Verification items for the finished model (mm, model axes). Round coordinates to 2 decimals unless told otherwise and drop trailing zeros. Write each loop counter-clockwise with the first axis right and the second up, starting at its lowest first coordinate (ties: lowest second). Pieces come first, ordered by that corner, then holes. Notation, with made-up numbers: M 77.5,68 L 83.5,68 A25 ccw 83.5,98 Z; hole C 43.25,-36 d4. An arc over 180 degrees is marked long. Use a Markdown table: item, result. Add a question column.
from build123d import *

# Parameters (mm, degrees)
ESQUISSE1_W             = 520
ESQUISSE1_H             = 42
BOSS_EXTRU_1_DEPTH      = 15
ESQUISSE2_R             = 10.5
ENL_V_MAT_EXTRU_1_DEPTH = 15
ESQUISSE3_W             = 10
ESQUISSE3_H             = 42
ENL_V_MAT_EXTRU_2_DEPTH = 262.277630118
ESQUISSE4_W             = 345
ESQUISSE4_H             = 5
ENL_V_MAT_EXTRU_3_DEPTH = 2


with BuildPart() as part:
    # Esquisse1 → Boss.-Extru.1 (new body)
    with BuildSketch(Plane(origin=(0, 0, 0), x_dir=(1, 0, 0), z_dir=(0, 1, 0))):
        Rectangle(ESQUISSE1_W, ESQUISSE1_H)
    extrude(amount=BOSS_EXTRU_1_DEPTH)

    # Esquisse2 → Enlèv. mat.-Extru.1 (cut)
    with BuildSketch(Plane(origin=(0, 15, 0), x_dir=(1, 0, 0), z_dir=(0, 1, 0))):
        with Locations(Location((-229, 0, 0), (0, 0, 270))):
            Circle(ESQUISSE2_R)
        with Locations(Location((229, 0, 0), (0, 0, 270))):
            Circle(ESQUISSE2_R)
    extrude(amount=-ENL_V_MAT_EXTRU_1_DEPTH, mode=Mode.SUBTRACT)

    # Esquisse3 → Enlèv. mat.-Extru.2 (cut, through all)
    with BuildSketch(Plane(origin=(0, 15, 0), x_dir=(1, 0, 0), z_dir=(0, 1, 0))):
        with Locations((-255, 0)):
            Rectangle(ESQUISSE3_W, ESQUISSE3_H)
        with Locations((255, 0)):
            Rectangle(ESQUISSE3_W, ESQUISSE3_H)
    extrude(amount=-ENL_V_MAT_EXTRU_2_DEPTH, mode=Mode.SUBTRACT)

    # Esquisse4 → Enlèv. mat.-Extru.3 (cut)
    with BuildSketch(Plane(origin=(0, 15, 0), x_dir=(1, 0, 0), z_dir=(0, 1, 0))):
        with Locations((-2.5, -10.5)):
            Rectangle(ESQUISSE4_W, ESQUISSE4_H)
        with Locations((-2.5, 10.5)):
            Rectangle(ESQUISSE4_W, ESQUISSE4_H)
    extrude(amount=-ENL_V_MAT_EXTRU_3_DEPTH, mode=Mode.SUBTRACT)


solid = part.part
1. Scan lines: line 1 along X through (y, z) = (9.25, 0); line 2 along X through (y, z) = (8.75, -7.5); line 3 along Y through (x, z) = (-105, -12). Record each from-to range of solid material in increasing order. Write a range as from..to.
2. Cross-section at C-C on y = 3.5. Enter the section's corners in (x, z), plus the area to 3 significant figures.
3. Cross-section at A-A on x = -229. Enter the section's corners in (y, z).
4. Release check for a two-part mould opening along Z. For faces 1 (the flat face through (-4, 7, -21)), 2 (the cylindrical face through (-218.59, 7.6, -1.37)), 3 (the flat face through (-4, 7, 21)) record: +Z half, -Z half, draft (parallel to the pull), parting line (faces both ways), or undercut.
5. Cross-section at B-B on z = 0. Enter the section's corners in (x, y), plus the area to 3 significant figures.
6. Depth check by flat-ended pin: pin 1 Ø1.5 at (x, z) = (-82.5, -11.5) entering from +Y. Enter the tip coordinate at first touch or a pass-through.
7. Cross-section at D-D on x = -92. Enter the section's corners in (y, z).
Answer:
| question | item | result |
|---|---|---|
| 1 | line 1 | x = -250..-239.5, -218.5..218.5, 239.5..250 |
| 1 | line 2 | x = -250..-236.35, -221.65..221.65, 236.35..250 |
| 1 | line 3 | y = 0..13 |
| 2 | outline | M -250,-21 L 250,-21 L 250,21 L -250,21 Z; hole C -229,0 d21; hole C 229,0 d21 |
| 2 | area | 20,300 mm^2 |
| 3 | outline | M 0,-21 L 15,-21 L 15,-10.5 L 0,-10.5 Z; M 0,10.5 L 15,10.5 L 15,21 L 0,21 Z |
| 4 | face 1 | -Z half |
| 4 | face 2 | undercut |
| 4 | face 3 | +Z half |
| 5 | outline | M -250,0 L -239.5,0 L -239.5,15 L -250,15 Z; M -218.5,0 L 218.5,0 L 218.5,15 L -218.5,15 Z; M 239.5,0 L 250,0 L 250,15 L 239.5,15 Z |
| 5 | area | 6,870 mm^2 |
| 6 | pin 1 | stops at y = 13 |
| 7 | outline | M 0,-21 L 15,-21 L 15,-13 L 13,-13 L 13,-8 L 15,-8 L 15,8 L 13,8 L 13,13 L 15,13 L 15,21 L 0,21 Z |
